from build123d import *

# Parameters (mm, degrees)
F0_W     = 172.72
F0_H     = 165.1
F0_W_2   = 25.104146
F0_H_2   = 4.064
F0_W_3   = 4.064
F0_H_3   = 33.9242
F0_W_4   = 24.795201
F0_W_5   = 21.220653
F0_H_4   = 44.69198
F0_W_6   = 35.56
F0_H_5   = 76.2
F0_H_6   = 34.7
F1_DEPTH = 5.08


with BuildPart() as f1:
    # F0 (on Top) → F1 (new body)
    with BuildSketch(Plane.XY):
        with Locations((0, -33.211574)):
            Rectangle(F0_W, F0_H)
        with Locations((-48.407927, -109.63035)):
            Rectangle(F0_W_2, F0_H_2, mode=Mode.SUBTRACT)
        with Locations((-80.213484, -84.063285)):
            Rectangle(F0_W_3, F0_H_3, mode=Mode.SUBTRACT)
        with Locations((1.941747, -109.63035)):
            Rectangle(F0_W_4, F0_H_2, mode=Mode.SUBTRACT)
        with Locations((50.349673, -109.63035)):
            Rectangle(F0_W_5, F0_H_2, mode=Mode.SUBTRACT)
        with Locations((80.213484, -84.063285)):
            Rectangle(F0_W_3, F0_H_3, mode=Mode.SUBTRACT)
        with Locations((-80.213484, -31.755195)):
            Rectangle(F0_W_3, F0_H_4, mode=Mode.SUBTRACT)
        with Locations((-55.88, -9.791071)):
            Rectangle(F0_W_6, F0_H_5, mode=Mode.SUBTRACT)
        with Locations((-80.213484, 27.940795)):
            Rectangle(F0_W_3, F0_H_6, mode=Mode.SUBTRACT)
        with Locations((-48.407927, 43.207203)):
            Rectangle(F0_W_2, F0_H_2, mode=Mode.SUBTRACT)
        with Locations((80.213484, -31.755195)):
            Rectangle(F0_W_3, F0_H_4, mode=Mode.SUBTRACT)
        with Locations((55.88, -9.791071)):
            Rectangle(F0_W_6, F0_H_5, mode=Mode.SUBTRACT)
        with Locations((1.941747, 43.207203)):
            Rectangle(F0_W_4, F0_H_2, mode=Mode.SUBTRACT)
        with Locations((80.213484, 27.940795)):
            Rectangle(F0_W_3, F0_H_6, mode=Mode.SUBTRACT)
        with Locations((50.349673, 43.207203)):
            Rectangle(F0_W_5, F0_H_2, mode=Mode.SUBTRACT)
    extrude(amount=F1_DEPTH)


solid = f1.part
Design review of the part built by this model. Coordinates are the model's own, in mm. A direction names the side the tool comes from. Round coordinates to 2 decimals unless told otherwise and drop trailing zeros. Write each loop counter-clockwise with the first axis right and the second up, starting at its lowest first coordinate (ties: lowest second). Pieces come first, ordered by that corner, then holes. Notation, with made-up numbers: (-31.75, 18) - (-7.75, 18) arc R25 cw to (-7.75, 33) - close; hole circle Ø4 at (77.25, 79). An arc over 180 degrees is marked (long way). Use a Markdown table: item, result. Add a question column.
1. We need section A-A (y = 20.5). State the section outline as (x, z) points.
2. Mouldability with a two-part tool opening along Y and no side actions: class faces 3 (the face through (86.36, -34, 3)), 4 (the face through (-82.245, -32, 3)), 5 (the face through (80, 10.591, 3)) as +Y half, -Y half, draft (parallel to the pull), parting line (faces both ways), or undercut.
3. We need section C-C (x = 66). State the section outline as (y, z) points.
4. We need section D-D (y = 0.5). State the section outline as (x, z) points, then the cut area to 3 significant figures.
5. We need section B-B (x = 46.5). State the section outline as (y, z) points.
6. Wall thickness on probe 1 along Y at (x, z) = (-45, 2.75); probe 2 along X at (y, z) = (-94, 4.6); probe 3 along X at (y, z) = (-44, 1.1): over which ranges is each line inside the solid? List them lowest first.
7. For faces 1 (the face through (-1, -50, 0)), 2 (the face through (2, -111.662, 3)), list the 3-axis set-ups (+Z, -Z, +X, -X, +Y, -Y) from which the entire face can be reached by the end or side of a thin tool; tool diameter is ignored.
Output:
| question | item | result |
|---|---|---|
| 1 | outline | (-86.36, 0) - (-82.25, 0) - (-82.25, 5.08) - (-86.36, 5.08) - close; (-78.18, 0) - (-73.66, 0) - (-73.66, 5.08) - (-78.18, 5.08) - close; (-38.1, 0) - (38.1, 0) - (38.1, 5.08) - (-38.1, 5.08) - close; (73.66, 0) - (78.18, 0) - (78.18, 5.08) - (73.66, 5.08) - close; (82.25, 0) - (86.36, 0) - (86.36, 5.08) - (82.25, 5.08) - close |
| 2 | face 3 | draft |
| 2 | face 4 | undercut |
| 2 | face 5 | undercut |
| 3 | outline | (-115.76, 0) - (-47.89, 0) - (-47.89, 5.08) - (-115.76, 5.08) - close; (28.31, 0) - (49.34, 0) - (49.34, 5.08) - (28.31, 5.08) - close |
| 4 | outline | (-86.36, 0) - (-73.66, 0) - (-73.66, 5.08) - (-86.36, 5.08) - close; (-38.1, 0) - (38.1, 0) - (38.1, 5.08) - (-38.1, 5.08) - close; (73.66, 0) - (86.36, 0) - (86.36, 5.08) - (73.66, 5.08) - close |
| 4 | area | 516 mm2 |
| 5 | outline | (-115.76, 0) - (-111.66, 0) - (-111.66, 5.08) - (-115.76, 5.08) - close; (-107.6, 0) - (-47.89, 0) - (-47.89, 5.08) - (-107.6, 5.08) - close; (28.31, 0) - (41.18, 0) - (41.18, 5.08) - (28.31, 5.08) - close; (45.24, 0) - (49.34, 0) - (49.34, 5.08) - (45.24, 5.08) - close |
| 6 | probe 1 | y = -115.76 to -111.66, -107.6 to -47.89, 28.31 to 41.18, 45.24 to 49.34 |
| 6 | probe 2 | x = -86.36 to -82.25, -78.18 to 78.18, 82.25 to 86.36 |
| 6 | probe 3 | x = -86.36 to -82.25, -78.18 to -73.66, -38.1 to 38.1, 73.66 to 78.18, 82.25 to 86.36 |
| 7 | face 1 | -Z, +X, -X, +Y, -Y |
| 7 | face 2 | +Z, -Z |
